from build123d import *

# Parameters (mm, degrees)
ESQUISSE1_W        = 4
ESQUISSE1_H        = 85
BOSS_EXTRU_1_DEPTH = 22.93
BOSS_EXTRU_5_DEPTH = 22.9
ESQUISSE5_W        = 25.35
ESQUISSE5_H        = 21.181614094
BOSS_EXTRU_6_DEPTH = 4
CONG_1_R           = 2
CONG_5_R           = 1
BOSS_EXTRU_8_DEPTH = 1
BOSS_EXTRU_9_DEPTH = 22.9


with BuildPart() as part:
    # Esquisse1 → Boss.-Extru.1 (new body)
    with BuildSketch(Plane.XY):
        with Locations((-2, -15.95097561)):
            Rectangle(ESQUISSE1_W, ESQUISSE1_H)
    extrude(amount=BOSS_EXTRU_1_DEPTH)

    # Esquisse2 → Boss.-Extru.5 (add)
    with BuildSketch(Plane.XY.offset(22.93)):
        Polygon((-33.850627534, 38.869645224), (0, 26.54902439), (0, 22.54902439), (-4, 22.54902439), (-35.604113867, 34.051981118), align=None)
    extrude(amount=-BOSS_EXTRU_5_DEPTH)

    # Esquisse5 → Boss.-Extru.6 (add)
    with BuildSketch(Plane.XY.offset(22.93)):
        with Locations((-12.675, -32.061782657)):
            Rectangle(ESQUISSE5_W, ESQUISSE5_H)
    extrude(amount=-BOSS_EXTRU_6_DEPTH)

    # Congé1
    cong_1_edges = [part.edges().sort_by_distance(p)[0] for p in [
        (-2, -58.45097561, 22.93),
        (-2, -58.45097561, 0),
    ]]
    fillet(cong_1_edges, radius=CONG_1_R)

    # Congé5
    cong_5_edges = [part.edges().sort_by_distance(p)[0] for p in [
        (-14.675, -21.47097561, 22.93),
        (-14.675, -42.652589704, 22.93),
    ]]
    fillet(cong_5_edges, radius=CONG_5_R)

    # Esquisse10 → Boss.-Extru.8 (add)
    with BuildSketch(Plane.ZY.offset(4)):
        with BuildLine():
            Line((10.166030362, 18.2390183), (11.166631323, 18.2390183))
            add(Edge.make_bspline(
                [(11.166631323, 18.2390183), (11.233404364, 18.238796034), (11.361615999, 18.238369259), (11.545292099, 18.235989598), (11.712187952, 18.22916909), (11.862216294, 18.223299685), (11.995374373, 18.212596912), (12.112070502, 18.202367416), (12.211767213, 18.188976472), (12.272118429, 18.176540153), (12.299443823, 18.170909326)],
                knots=[0, 0, 0, 0, 0.000200323, 0.000384642, 0.000551017, 0.000701421, 0.00083501, 0.000951717, 0.001052854, 0.001136534, 0.001136534, 0.001136534, 0.001136534], degree=3))
            add(Edge.make_bspline(
                [(12.299443823, 18.170909326), (12.336024715, 18.161871089), (12.408406128, 18.143987427), (12.512620508, 18.106187997), (12.611926685, 18.062445676), (12.705912149, 18.011068933), (12.794106136, 17.951676391), (12.877418009, 17.885293359), (12.956225814, 17.812283065), (13.027342428, 17.73080472), (13.094398216, 17.645323991), (13.150953397, 17.552890053), (13.199705511, 17.456230728), (13.238520535, 17.354362988), (13.269774783, 17.248274743), (13.291812268, 17.137005033), (13.30502825, 17.021060783), (13.306373758, 16.941978056), (13.307056003, 16.901878877)],
                knots=[0, 0, 0, 0, 0.000112973, 0.000223535, 0.000332046, 0.000438282, 0.0005444, 0.000650613, 0.000757615, 0.000866163, 0.000974744, 0.001083144, 0.001190647, 0.001299089, 0.001409706, 0.001522064, 0.001638977, 0.001759236, 0.001759236, 0.001759236, 0.001759236], degree=3))
            add(Edge.make_bspline(
                [(13.307056003, 16.901878877), (13.304957434, 16.835257299), (13.300862583, 16.705261345), (13.262683863, 16.516602943), (13.200145978, 16.340618207), (13.113969851, 16.177528725), (13.004227743, 16.030513517), (12.872335184, 15.901384295), (12.718218596, 15.793327277), (12.574748145, 15.718394699), (12.448013574, 15.67040483), (12.34368027, 15.636638603), (12.229870302, 15.610550081), (12.10767411, 15.587178464), (11.976583173, 15.569533186), (11.836911688, 15.55660948), (11.688560043, 15.548532268), (11.586647087, 15.547329403), (11.534219464, 15.546710608)],
                knots=[0, 0, 0, 0, 0.000199681, 0.000389629, 0.000574641, 0.000758347, 0.00094084, 0.00112287, 0.00130963, 0.001503603, 0.001606651, 0.001715936, 0.001832303, 0.001956651, 0.002089094, 0.002228924, 0.002377378, 0.002534658, 0.002534658, 0.002534658, 0.002534658], degree=3))
            Line((11.534219464, 15.546710608), (13.371158567, 13.2390183))
            Line((13.371158567, 13.2390183), (12.816270746, 13.2390183))
            Line((12.816270746, 13.2390183), (10.979331644, 15.546710608))
            Line((10.979331644, 15.546710608), (10.61474831, 15.546710608))
            Line((10.61474831, 15.546710608), (10.61474831, 13.2390183))
            Line((10.61474831, 13.2390183), (10.166030362, 13.2390183))
            Line((10.166030362, 13.2390183), (10.166030362, 18.2390183))
        make_face()
        with BuildLine():
            Line((10.61474831, 17.726197787), (10.61474831, 16.05953112))
            Line((10.61474831, 16.05953112), (11.530213054, 16.052519902))
            add(Edge.make_bspline(
                [(11.530213054, 16.052519902), (11.572955967, 16.052500993), (11.655803905, 16.052464341), (11.775661998, 16.058169736), (11.887262158, 16.06466019), (11.990177518, 16.074587827), (12.084454054, 16.087382215), (12.170044644, 16.103386478), (12.247089004, 16.122032282), (12.336944059, 16.150891747), (12.437281961, 16.196614631), (12.546326904, 16.263136772), (12.639187386, 16.346806942), (12.717641475, 16.442483308), (12.78068352, 16.547677949), (12.825129312, 16.661129905), (12.853332801, 16.779975045), (12.856659294, 16.861658056), (12.858338054, 16.902880479)],
                knots=[0, 0, 0, 0, 0.000128209, 0.000248506, 0.000359904, 0.000463555, 0.000558601, 0.000645233, 0.000724669, 0.000796254, 0.000928055, 0.001054503, 0.00117794, 0.001301056, 0.001424562, 0.001544156, 0.0016654, 0.001788926, 0.001788926, 0.001788926, 0.001788926], degree=3))
            add(Edge.make_bspline(
                [(12.858338054, 16.902880479), (12.856620738, 16.94308987), (12.853217645, 17.022770211), (12.82543369, 17.139421512), (12.778448859, 17.249517155), (12.715131376, 17.352609276), (12.637989726, 17.446188899), (12.547535708, 17.52625626), (12.446242572, 17.592326924), (12.351569432, 17.634547468), (12.266949128, 17.660432973), (12.193478185, 17.678648921), (12.110461789, 17.693283876), (12.017496848, 17.705009678), (11.914980232, 17.715088169), (11.802393588, 17.721876425), (11.680483902, 17.725896231), (11.595988286, 17.726094929), (11.55224831, 17.726197787)],
                knots=[0, 0, 0, 0, 0.00012053, 0.000238846, 0.000357345, 0.000478278, 0.000600621, 0.000719816, 0.000839275, 0.000962126, 0.001029286, 0.001104593, 0.001189072, 0.001282, 0.00138565, 0.001498049, 0.00162031, 0.001751524, 0.001751524, 0.001751524, 0.001751524], degree=3))
            Line((11.55224831, 17.726197787), (10.61474831, 17.726197787))
        make_face(mode=Mode.SUBTRACT)
    extrude(amount=BOSS_EXTRU_8_DEPTH)

    # Esquisse11 → Boss.-Extru.9 (add)
    with BuildSketch(Plane.XY.offset(22.93)):
        Polygon((-5.452843765, 23.077816276), (-4, 20.298440223), (-0.659211444, 23.077816276), align=None)
    extrude(amount=-BOSS_EXTRU_9_DEPTH)


solid = part.part
CAD build for the part. Positions are in the model's coordinates, mm. A direction names the side the tool comes from. Coordinates: 2 decimals unless noted, no trailing zeros. Order: outer loops, then holes, each group sorted by start corner. A loop starts at its lowest first (then second) coordinate and runs counter-clockwise, first axis right, second up.
Item 1: Band-saw the part on D-D on y = -16. List the corners of the cut face in (x, z).
Check sheet entries:
outline: (-4, 0) - (0, 0) - (0, 22.93) - (-4, 22.93) - close
Item 2: Pin check, flat tips, straight feed: pin 1 Ø1.5 at (x, z) = (-24.5, 3) entering from -Y; pin 2 Ø0.5 at (x, y) = (-4.5, 15.5) entering from -Z; pin 3 Ø6 at (y, z) = (-33, 15.5) entering from +X; pin 4 Ø1.6 at (y, z) = (17, 11) entering from -X. Stop position of each tip, or through.
Check sheet entries:
pin 1: stops at y = 29.74
pin 2: stops at z = 10.17
pin 3: stops at x = 0
pin 4: stops at x = -5
Item 3: Band-saw the part on A-A on x = -11. List the corners of the cut face in (y, z).
Check sheet entries:
outline: (-42.65, 18.93) - (-21.47, 18.93) - (-21.47, 21.93) arc R1 ccw to (-22.47, 22.93) - (-41.65, 22.93) arc R1 ccw to (-42.65, 21.93) - close; (25.1, 0.03) - (30.55, 0.03) - (30.55, 22.93) - (25.1, 22.93) - close
Item 4: Two-plate mould, pull along Z, no slides. Class faces 1 (the face through (-1.97, -57.88, 0.6)), 2 (the face through (-4.49, 14.38, 11.91)), 3 (the face through (-4, 17, 12)), 4 (the face through (-20.32, 28.49, 11.64)): +Z half, -Z half, draft (parallel to the pull), parting line (faces both ways), or undercut.
Check sheet entries:
face 1: -Z half
face 2: undercut
face 3: undercut
face 4: draft
Item 5: Band-saw the part on B-B on y = -28.5. List the corners of the cut face in (x, z), plus the area to 3 significant figures.
Check sheet entries:
outline: (-25.35, 18.93) - (-4, 18.93) - (-4, 0) - (0, 0) - (0, 22.93) - (-25.35, 22.93) - close
area: 177 mm2
Item 6: 3-axis set-ups, long thin cutter, end or side, ignore diameter. For faces 5 (the face through (-15, -21.471, 20)), 6 (the face through (-15, -32, 18.93)), 7 (the face through (-34.74, 36.43, 11.64)), 8 (the face through (-15, -42.653, 20)): which of +Z, -Z, +X, -X, +Y, -Y reach the whole face in a straight line?
Check sheet entries:
face 5: +Z, -Z, -X
face 6: -Z, -X, -Y
face 7: +Z, -Z, -X, +Y
face 8: +Z, -Z, -X, -Y
Item 7: Drill centre lines: L1, parallel to X at y = -53, z = 12.75; L2, parallel to Z at x = -10.5, y = -27; L3, parallel to Y at x = -23.5, z = 19.75. Where is each one in solid material? Low to high.
Check sheet entries:
L1: x = -4 to 0
L2: z = 18.93 to 22.93
L3: y = -42.65 to -21.47, 29.65 to 35.1
Item 8: Band-saw the part on C-C on z = 3. List the corners of the cut face in (x, y), plus the area to 3 significant figures.
Check sheet entries:
outline: (-35.6, 34.05) - (-5.45, 23.08) - (-4, 20.3) - (-4, -58.45) - (0, -58.45) - (0, 26.55) - (-33.85, 38.87) - close
area: 512 mm2
